Autodesk Inventor part; units mm, degrees
ref_plane "YZ Plane" through (0, 0, 0) normal (1, 0, 0) x (0, 1, 0)
ref_plane "XZ Plane" through (0, 0, 0) normal (0, 1, 0) x (-1, 0, 0)
ref_plane "XY Plane" through (0, 0, 0) normal (0, 0, 1) x (1, 0, 0)
sketch "Эскиз1" plane through (0, 0, 0) normal (0, 0, 1) x (1, 0, 0)
  line L0 (-18.25, -37.6) -> (18.25, -37.6)
  line L1 (18.25, -37.6) -> (18.25, 37.6)
  line L2 (18.25, 37.6) -> (-18.25, 37.6)
  line L3 (-18.25, 37.6) -> (-18.25, -37.6)
  line L4 (-18.25, 0) -> (18.25, 0) construction
  line L5 (0, 37.6) -> (0, -37.6) construction
  line L6 (-18.45, -37.8) -> (18.45, -37.8)
  line L7 (18.45, -37.8) -> (18.45, 37.8)
  line L8 (18.45, 37.8) -> (-18.45, 37.8)
  line L9 (-18.45, 37.8) -> (-18.45, -37.8)
  line L10 (-7.5, -37.8) -> (7.5, -37.8)
  line L11 (7.5, -37.8) -> (7.5, -40.8)
  line L12 (7.5, -40.8) -> (-7.5, -40.8)
  line L13 (-7.5, -40.8) -> (-7.5, -37.8)
  line L14 (-18.45, -37.8) -> (-18.45, -43.8)
  line L15 (-18.45, -43.8) -> (18.45, -43.8)
  line L16 (18.45, -43.8) -> (18.45, -37.8)
  line L17 (-18.45, 37.8) -> (-18.45, 43.8)
  line L18 (-18.45, 43.8) -> (18.45, 43.8)
  line L19 (18.45, 43.8) -> (18.45, 37.8)
  line L20 (-18.45, -43.8) -> (-21.45, -43.8)
  line L21 (-21.45, -43.8) -> (-21.45, 43.8)
  line L22 (-21.45, 43.8) -> (-18.45, 43.8)
  line L23 (-18.45, 43.8) -> (-18.45, -43.8)
  line L24 (18.45, 37.8) -> (18.45, 43.8)
  line L25 (21.45, -43.8) -> (21.45, 43.8)
  line L26 (21.45, 43.8) -> (18.45, 43.8)
  line L27 (18.45, 43.8) -> (18.45, -43.8)
  line L28 (7.5, 37.8) -> (7.5, 40.8)
  line L29 (7.5, 40.8) -> (-7.5, 40.8)
  line L30 (-7.5, 40.8) -> (-7.5, 37.8)
  line L31 (-21.45, -43.8) -> (-11.45, -43.8)
  line L32 (18.45, -43.8) -> (21.45, -43.8)
  line L33 (21.45, -43.8) -> (11.45, -43.8)
  line L34 (16.45, 46.7) -> (21.45, 46.7)
  line L35 (16.45, 46.7) -> (11.45, 46.7)
  line L36 (11.45, 46.7) -> (11.45, 43.8)
  line L37 (21.45, 46.7) -> (21.45, 43.8)
  line L38 (11.45, 43.8) -> (16.45, 43.8)
  circle A0 centre (16.45, 43.8) radius 2.1
  line L39 (-16.45, 46.7) -> (-21.45, 46.7)
  line L40 (-16.45, 46.7) -> (-11.45, 46.7)
  line L41 (-11.45, 46.7) -> (-11.45, 43.8)
  line L42 (-21.45, 46.7) -> (-21.45, 43.8)
  circle A1 centre (-16.45, 43.8) radius 2.1
  line L43 (16.45, -46.7) -> (21.45, -46.7)
  line L44 (16.45, -46.7) -> (11.45, -46.7)
  line L45 (11.45, -46.7) -> (11.45, -43.8)
  line L46 (21.45, -46.7) -> (21.45, -43.8)
  circle A2 centre (16.45, -43.8) radius 2.1
  line L47 (-11.45, -46.7) -> (-11.45, -43.8)
  line L48 (-16.45, -46.7) -> (-11.45, -46.7)
  line L49 (-16.45, -46.7) -> (-21.45, -46.7)
  line L50 (-21.45, -46.7) -> (-21.45, -43.8)
  circle A3 centre (-16.45, -43.8) radius 2.1
  point P0 (0, 0)
  point P1 (0, 0)
  point P2 (-1.9914, -32.8601)
  point P3 (0, -37.8)
  dimension "d0" = 36.5
  dimension "d1" = 75.2
  dimension "d4" = 36.9
  dimension "d5" = 75.6
  dimension "d6" = 15
  dimension "d7" = 3
  dimension "d9" = 6
  dimension "d10" = 3
  dimension "d18" = 5
  dimension "d19" = 4.2
extrude "Выдавливание1" add sketch "Эскиз1" along normal blind 25 contours L14 A3 L20 L21 L22 A1 L17 L9 | L6 L13 L12 L11 L16 A2 L15 A3 L14 | L6 L11 L12 L13 | L17 A1 L18 A0 L19 L8 L28 L29 L30 | A3 L15 L14 | L14 L20 A3 | L30 L29 L28 L8 | A1 L22 L17 | L17 L18 A1 | L15 A3 L20 | L15 L47 L48 L49 L50 L20 A3 | L7 L19 A0 L26 L25 L32 A2 L16 | L22 A1 L18 | L22 L42 L39 L40 L41 L18 A1 | A2 L32 L16 | L16 L15 A2 | L15 A2 L32 L46 L43 L44 L45 | A0 L18 L19 | L19 L26 A0 | L32 A2 L15 | L36 L35 L34 L37 L26 A0 L18 | L18 A0 L26
extrude "Выдавливание2" cut sketch "Эскиз1" along normal blind 8 contours A3 L15 L14 | L14 L20 A3 | A1 L22 L17 | L17 L18 A1 | L15 A3 L20 | L22 A1 L18 | A2 L32 L16 | L16 L15 A2 | A0 L18 L19 | L19 L26 A0 | L32 A2 L15 | L18 A0 L26
extrude "Выдавливание3" cut sketch "Эскиз1" along normal blind 22.5 contours L6 L11 L12 L13 | L30 L29 L28 L8
fillet "Сопряжение1" radius 2 4 edges at (21.45, -46.7, 12.5) (-21.45, -46.7, 12.5) (-21.45, 46.7, 12.5) (21.45, 46.7, 12.5)
properties part number "fast_akkum"
Read the model definition and answer for the solid it produces. Units are mm, in the model's axes. A direction names the side the tool comes from. Give positions to 0.01 mm unless a question says otherwise; leave off trailing zeros. Loops run counter-clockwise (first coordinate to the right, second up) from the corner with the lowest first, then second, coordinate; pieces in that order, holes last. Notation, with made-up numbers: (4, 61) -> (29, 61) arc R12 ccw to (29, 68) -> close; hole circle Ø9 at (44.5, 35). An arc over 180 degrees is marked (long way). Use a Markdown table: item, result.
Q1. Section B-B, the plane y = 10 is taken. Determine the outline of the cut face in (x, z), then the cut area to 3 significant figures.
Solved:
| item | result |
|---|---|
| outline | (-21.45, 0) -> (-18.45, 0) -> (-18.45, 25) -> (-21.45, 25) -> close; (18.45, 0) -> (21.45, 0) -> (21.45, 25) -> (18.45, 25) -> close |
| area | 150 mm^2 |
Q2. Section D-D, the plane z = 20.25 is taken. Determine the outline of the cut face in (x, y), then the cut area to 3 significant figures.
Solved:
| item | result |
|---|---|
| outline | (-21.45, -44.7) arc R2 ccw to (-19.45, -46.7) -> (-11.45, -46.7) -> (-11.45, -43.8) -> (11.45, -43.8) -> (11.45, -46.7) -> (19.45, -46.7) arc R2 ccw to (21.45, -44.7) -> (21.45, 44.7) arc R2 ccw to (19.45, 46.7) -> (11.45, 46.7) -> (11.45, 43.8) -> (-11.45, 43.8) -> (-11.45, 46.7) -> (-19.45, 46.7) arc R2 ccw to (-21.45, 44.7) -> close; hole (-18.45, -37.8) -> (-7.5, -37.8) -> (-7.5, -40.8) -> (7.5, -40.8) -> (7.5, -37.8) -> (18.45, -37.8) -> (18.45, 37.8) -> (7.5, 37.8) -> (7.5, 40.8) -> (-7.5, 40.8) -> (-7.5, 37.8) -> (-18.45, 37.8) -> close |
| area | 991 mm^2 |
Q3. Determine the mould class of faces 4 (the face through (-15, 46.7, 12)), 5 (the face through (15.99, 45.85, 3.94)), 6 (the face through (0, -43.8, 12)) for opening direction Y: pulls with the +Y half, pulls with the -Y half, needs draft (parallel to the pull), parting line crosses it, or undercut.
Solved:
| item | result |
|---|---|
| face 4 | pulls with the +Y half |
| face 5 | undercut |
| face 6 | pulls with the -Y half |
Q4. A tool of negligible diameter and unlimited length cuts with its end or side. For faces 1 (the face through (11.45, -45, 12)), 2 (the face through (0, 43.8, 12)), 3 (the face through (0, 40.8, 11)), from which of +Z, -Z, +X, -X, +Y, -Y can it reach the whole face along a straight path? Write none if from no direction.
Solved:
| item | result |
|---|---|
| face 1 | +Z, -Z, -Y |
| face 2 | +Z, -Z, +Y |
| face 3 | -Z |
Q5. Section C-C, the plane z = 3.25 is taken. Count the separate pieces of the cut face and the enclosed holes in it, then the cut area to 3 significant figures.
Solved:
| item | result |
|---|---|
| separate pieces | 1 |
| enclosed holes | 5 |
| area | 936 mm^2 |
Q6. Each of these flat-tipped pins is pushed along its axis until it touches: pin 1 (12 mm diameter, centred on x = 0, z = 10, fed in from -Y); pin 2 (3 mm diameter, centred on x = 8, z = 4.5, fed in from +Y); pin 3 (1.3 mm diameter, centred on x = -16, y = -44, fed in from -Z). Where does it stop, or does it pass through?
Solved:
| item | result |
|---|---|
| pin 1 | stops at y = -43.8 |
| pin 2 | stops at y = 43.8 |
| pin 3 | stops at z = 8 |
Q7. Find the intervals of material crossed by line 1 along Y through (x, z) = (16.45, 6.5); line 2 along X through (y, z) = (-19.5, 7.75); line 3 along Y through (x, z) = (11.5, 18.25), in increasing order.
Solved:
| item | result |
|---|---|
| line 1 | y = -46.7 to -45.9, -41.7 to -37.8, 37.8 to 41.7, 45.9 to 46.7 |
| line 2 | x = -21.45 to -18.45, 18.45 to 21.45 |
| line 3 | y = -46.7 to -37.8, 37.8 to 46.7 |
Q8. Section A-A, the plane x = 16.45 is taken. Determine the outline of the cut face in (y, z).
Solved:
| item | result |
|---|---|
| outline | (-46.7, 0) -> (-45.9, 0) -> (-45.9, 8) -> (-41.7, 8) -> (-41.7, 0) -> (-37.8, 0) -> (-37.8, 25) -> (-46.7, 25) -> close; (37.8, 0) -> (41.7, 0) -> (41.7, 8) -> (45.9, 8) -> (45.9, 0) -> (46.7, 0) -> (46.7, 25) -> (37.8, 25) -> close |
